```python
from build123d import *

# Parameters (mm, degrees)
F0_W     = 50
F0_H     = 80
F1_DEPTH = 4
F2_W     = 4
F2_H     = 3.5
F3_DEPTH = 50.001
F4_R     = 1
F5_DEPTH = 4
F6_R     = 1
F7_DEPTH = 4
F8_R     = 1
F9_DEPTH = 4


with BuildPart() as f1:
    # F0 (on Right) → F1 (new body, symmetric)
    with BuildSketch(Plane.YZ):
        Rectangle(F0_W, F0_H)
    extrude(amount=F1_DEPTH, both=True)

    # F2 (on face) → F3 (cut, through all)
    with BuildSketch(Plane.XZ.offset(25)):
        with Locations((2, 38.25)):
            Rectangle(F2_W, F2_H)
        with Locations((2, -10.25)):
            Rectangle(F2_W, F2_H)
        with Locations((2, -38.25)):
            Rectangle(F2_W, F2_H)
    extrude(amount=-F3_DEPTH, mode=Mode.SUBTRACT)

    # F4 (on face) → F5 (cut, through all)
    with BuildSketch(Plane.YZ):
        with Locations((-15, 38.25)):
            Circle(F4_R)
        with Locations((15, 38.25)):
            Circle(F4_R)
    extrude(amount=-F5_DEPTH, mode=Mode.SUBTRACT)

    # F6 (on face) → F7 (cut, through all)
    with BuildSketch(Plane.YZ):
        with Locations((-15, -10.25)):
            Circle(F6_R)
        with Locations((15, -10.25)):
            Circle(F6_R)
    extrude(amount=-F7_DEPTH, mode=Mode.SUBTRACT)

    # F8 (on face) → F9 (cut, through all)
    with BuildSketch(Plane.YZ):
        with Locations((-15, -38.25)):
            Circle(F8_R)
        with Locations((15, -38.25)):
            Circle(F8_R)
    extrude(amount=-F9_DEPTH, mode=Mode.SUBTRACT)


solid = f1.part
```
Could you check a few things on this model? Use its own coordinates, in mm. A direction names the side the tool comes from. Coordinates: 2 decimals unless noted, no trailing zeros. Loops run counter-clockwise (first coordinate to the right, second up) from the corner with the lowest first, then second, coordinate; pieces in that order, holes last.
1) Imagine slicing it at A-A (x = 1.5). List the corners of the cut face in (y, z) for me.
Reported:
outline: (-25, -36.5) - (25, -36.5) - (25, -12) - (-25, -12) - close; (-25, -8.5) - (25, -8.5) - (25, 36.5) - (-25, 36.5) - close
2) Which directions (+Z, -Z, +X, -X, +Y, -Y) give clear straight access to the entire face, cutting with the end or side of a thin tool? Please do faces 4 (the face through (-4, 0, 1)), 5 (the face through (-2, 0, -40)), 6 (the face through (0, 0, -10)), 7 (the face through (2, 0, -36.5)), 8 (the face through (2, 0, 36.5)).
Reported:
face 4: +Z, -Z, -X, +Y, -Y
face 5: -Z, +X, -X, +Y, -Y
face 6: +X, +Y, -Y
face 7: -Z, +X, +Y, -Y
face 8: +Z, +X, +Y, -Y
3) Will these pins go through, and if not, where does the flat tip stop? pin 1 Ø1.6 at (y, z) = (-15, -38.25) entering from +X; pin 2 Ø2.5 at (y, z) = (-15, -10.25) entering from +X; pin 3 Ø1.2 at (x, y) = (1.5, -12) entering from -Z; pin 4 Ø2 at (x, y) = (2.5, 5.5) entering from +Z.
Reported:
pin 1: passes through
pin 2: stops at x = 0
pin 3: stops at z = -36.5
pin 4: stops at z = 36.5
4) Imagine slicing it at B-B (z = 38.25). List the corners of the cut face in (x, y) for me.
Reported:
outline: (-4, -25) - (0, -25) - (0, -16) - (-4, -16) - close; (-4, -14) - (0, -14) - (0, 14) - (-4, 14) - close; (-4, 16) - (0, 16) - (0, 25) - (-4, 25) - close
5) Thinking about a two-plate mould opening in Y: for faces 1 (the face through (0, 0, 38)), 2 (the face through (-1.97, -14.46, 39.09)), 3 (the face through (0, -25, -1)), which applies, released by +Y, released by -Y, zero draft, split by the parting line, or undercut?
Reported:
face 1: zero draft
face 2: undercut
face 3: released by -Y
6) Please list where these lines run through material, in increasing order: line 1 along Z through (x, y) = (-1.9, -15); line 2 along Z through (x, y) = (1.5, 11).
Reported:
line 1: z = -40 to -39.25, -37.25 to -11.25, -9.25 to 37.25, 39.25 to 40
line 2: z = -36.5 to -12, -8.5 to 36.5
7) Imagine slicing it at C-C (y = 15). List the corners of the cut face in (x, z) for me.
Reported:
outline: (-4, -40) - (0, -40) - (0, -39.25) - (-4, -39.25) - close; (-4, -37.25) - (0, -37.25) - (0, -36.5) - (4, -36.5) - (4, -12) - (0, -12) - (0, -11.25) - (-4, -11.25) - close; (-4, -9.25) - (0, -9.25) - (0, -8.5) - (4, -8.5) - (4, 36.5) - (0, 36.5) - (0, 37.25) - (-4, 37.25) - close; (-4, 39.25) - (0, 39.25) - (0, 40) - (-4, 40) - close
8) Imagine slicing it at D-D (y = 5.5). List the corners of the cut face in (x, z) for me.
Reported:
outline: (-4, -40) - (0, -40) - (0, -36.5) - (4, -36.5) - (4, -12) - (0, -12) - (0, -8.5) - (4, -8.5) - (4, 36.5) - (0, 36.5) - (0, 40) - (-4, 40) - close
